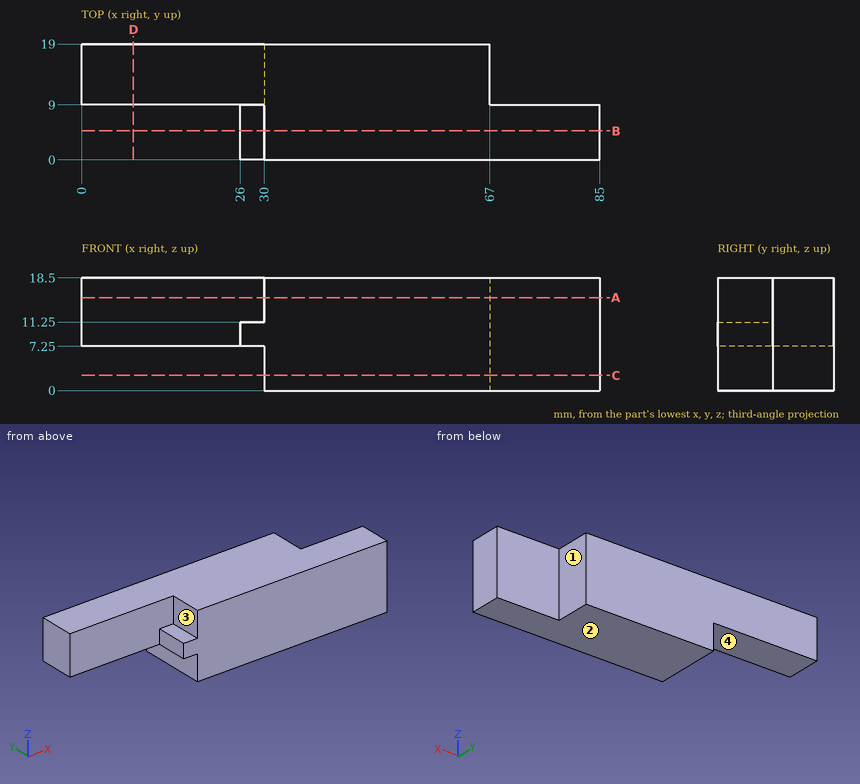
Input: dimensioned drawing with shaded views. Units: mm. Origin: part minimum x, y, z. A direction names the side the tool comes from. Coordinates: 2 decimals unless noted, no trailing zeros. Loops run counter-clockwise (first coordinate to the right, second up) from the corner with the lowest first, then second, coordinate; pieces in that order, holes last. Notation, with made-up numbers: (-18.5, -17) -> (33.5, -17) arc R28 ccw to (33.5, 3) -> close; hole circle Ø8 at (-38, 82). An arc over 180 degrees is marked (long way). Use a Markdown table: item, result. Add a question column.
(1) Line query: line 1 along X through (y, z) = (10.25, 16.5); line 2 along X through (y, z) = (9.75, 6.5); line 3 along Z through (x, y) = (23, 14.5). Output: solid intervals per line, ascending.
(2) Section query D-D, the plane x = 8.5. Return loops of the section in (y, z).
(3) Section query C-C, the plane z = 2.5. Return loops of the section in (x, y), plus the area to 3 significant figures.
(4) Section query A-A, the plane z = 15.25. Return loops of the section in (x, y), plus the area to 4 significant figures.
(5) Section query B-B, the plane y = 4.75. Return loops of the section in (x, z).
(6) Pin query (flat end, axial travel): pin 1 Ø3.5 at (y, z) = (12.5, 4) entering from -X; pin 2 Ø5 at (x, z) = (14.5, 14.5) entering from -Y; pin 3 Ø5 at (y, z) = (13.5, 12) entering from +X. Return the tip coordinate at first contact, or that it passes through.
(7) Access query for the marked faces 1, 2, 3 and 4. Directions: +Z, -Z, +X, -X, +Y, -Y. A direction counts if a zero-diameter tool reaches every point of the face in a straight line with its end or side. Return the directions, or none.
Answer:
| question | item | result |
|---|---|---|
| 1 | line 1 | x = 0 to 67 |
| 1 | line 2 | x = 30 to 67 |
| 1 | line 3 | z = 7.25 to 18.5 |
| 2 | outline | (9, 7.25) -> (19, 7.25) -> (19, 18.5) -> (9, 18.5) -> close |
| 3 | outline | (30, 0) -> (85, 0) -> (85, 9) -> (67, 9) -> (67, 19) -> (30, 19) -> close |
| 3 | area | 865 mm^2 |
| 4 | outline | (0, 9) -> (30, 9) -> (30, 0) -> (85, 0) -> (85, 9) -> (67, 9) -> (67, 19) -> (0, 19) -> close |
| 4 | area | 1,165 mm^2 |
| 5 | outline | (26, 7.25) -> (30, 7.25) -> (30, 0) -> (85, 0) -> (85, 18.5) -> (30, 18.5) -> (30, 11.25) -> (26, 11.25) -> close |
| 6 | pin 1 | stops at x = 30 |
| 6 | pin 2 | stops at y = 9 |
| 6 | pin 3 | stops at x = 67 |
| 7 | face 1 | +Z, -Z, +X, +Y |
| 7 | face 2 | -Z, +X, -X, +Y, -Y |
| 7 | face 3 | +Z, -X, -Y |
| 7 | face 4 | -Z, -X, +Y, -Y |
